Could you check a few things on this model? Use its own coordinates, in mm. Face numbers are marked on the shaded views. A direction names the side the tool comes from. Coordinates: 2 decimals unless noted, no trailing zeros. Loops run counter-clockwise (first coordinate to the right, second up) from the corner with the lowest first, then second, coordinate; pieces in that order, holes last. Notation, with made-up numbers: (-31.5, -31) - (-11.5, -31) arc R26 ccw to (-11.5, -13) - close; hole circle Ø2 at (10, 87.25). An arc over 180 degrees is marked (long way). Put each result on its own line as item: value. Start each with the question number.
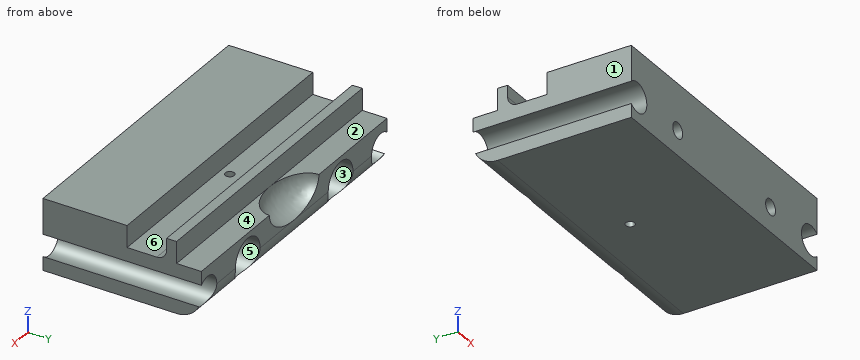
```python
from build123d import *

# Parameters (mm, degrees)
SKETCH2_W           = 18.288
SKETCH2_H           = 40.64
BOSS_EXTRUDE1_DEPTH = 76.2
CUT_EXTRUDE1_REACH  = 90.275
SKETCH3_W           = 5.588
SKETCH3_H           = 6.35
SKETCH3_H_2         = 10.16
CUT_EXTRUDE2_REACH  = 89.289
SKETCH4_R           = 1.143
CUT_EXTRUDE3_REACH  = 90.275
SKETCH5_R           = 2.032
SKETCH6_R           = 5.08
CUT_EXTRUDE4_DEPTH  = 15.24
FILLET1_R           = 6.35
FILLET2_R           = 2.54
SKETCH7_R           = 3.81
CUT_EXTRUDE5_DEPTH  = 89.275141297


with BuildPart() as part:
    # Sketch2 → Boss-Extrude1 (new body)
    with BuildSketch(Plane(origin=(0, 0, 0), x_dir=(0, 0, -1), z_dir=(1, 0, 0))):
        with Locations((9.144, 20.32)):
            Rectangle(SKETCH2_W, SKETCH2_H)
    extrude(amount=BOSS_EXTRUDE1_DEPTH)

    # Sketch3 → Cut-Extrude1 (cut, up to next)
    with BuildSketch(Plane.ZY, mode=Mode.PRIVATE) as cut_extrude1_sk1:
        with Locations((-2.794, 37.465)):
            Rectangle(SKETCH3_W, SKETCH3_H)
    cut_extrude1_tool1 = extrude(cut_extrude1_sk1.sketch, amount=-CUT_EXTRUDE1_REACH, mode=Mode.PRIVATE) & part.part
    # Sketch3 → Cut-Extrude1 (cut, up to next)
    with BuildSketch(Plane.ZY, mode=Mode.PRIVATE) as cut_extrude1_sk2:
        with Locations((-2.794, 26.67)):
            Rectangle(SKETCH3_W, SKETCH3_H_2)
    cut_extrude1_tool2 = extrude(cut_extrude1_sk2.sketch, amount=-CUT_EXTRUDE1_REACH, mode=Mode.PRIVATE) & part.part
    add(cut_extrude1_tool1.solids().sort_by_distance((0, 37.465, -2.794))[0], mode=Mode.SUBTRACT)
    add(cut_extrude1_tool2.solids().sort_by_distance((0, 26.67, -2.794))[0], mode=Mode.SUBTRACT)

    # Sketch4 → Cut-Extrude2 (cut, up to next)
    with BuildSketch(Plane.XY.offset(-5.588), mode=Mode.PRIVATE) as cut_extrude2_sk1:
        with Locations((38.1, 24.13)):
            Circle(SKETCH4_R)
    cut_extrude2_tool1 = extrude(cut_extrude2_sk1.sketch, amount=-CUT_EXTRUDE2_REACH, mode=Mode.PRIVATE) & part.part
    add(cut_extrude2_tool1.solids().sort_by_distance((38.1, 24.13, -5.588))[0], mode=Mode.SUBTRACT)

    # Sketch5 → Cut-Extrude3 (cut, up to next)
    with BuildSketch(Plane(origin=(0, 40.64, 0), x_dir=(1, 0, 0), z_dir=(0, 1, 0)), mode=Mode.PRIVATE) as cut_extrude3_sk1:
        with Locations(Location((57.15, 11.938, 0), (0, 0, 270))):
            Circle(SKETCH5_R)
    cut_extrude3_tool1 = extrude(cut_extrude3_sk1.sketch, amount=-CUT_EXTRUDE3_REACH, mode=Mode.PRIVATE) & part.part
    # Sketch5 → Cut-Extrude3 (cut, up to next)
    with BuildSketch(Plane(origin=(0, 40.64, 0), x_dir=(1, 0, 0), z_dir=(0, 1, 0)), mode=Mode.PRIVATE) as cut_extrude3_sk2:
        with Locations(Location((19.05, 11.938, 0), (0, 0, 270))):
            Circle(SKETCH5_R)
    cut_extrude3_tool2 = extrude(cut_extrude3_sk2.sketch, amount=-CUT_EXTRUDE3_REACH, mode=Mode.PRIVATE) & part.part
    add(cut_extrude3_tool1.solids().sort_by_distance((57.15, 40.64, -11.938))[0], mode=Mode.SUBTRACT)
    add(cut_extrude3_tool2.solids().sort_by_distance((19.05, 40.64, -11.938))[0], mode=Mode.SUBTRACT)

    # Sketch6 → Cut-Extrude4 (cut)
    with BuildSketch(Plane(origin=(0, 40.64, 0), x_dir=(1, 0, 0), z_dir=(0, 1, 0))):
        with Locations(Location((19.05, 11.938, 0), (0, 0, 270))):
            Circle(SKETCH6_R)
        with Locations(Location((57.15, 11.938, 0), (0, 0, 270))):
            Circle(SKETCH6_R)
    extrude(amount=-CUT_EXTRUDE4_DEPTH, mode=Mode.SUBTRACT)

    # Fillet1
    # the kernel refuses this fillet: 6.35 mm, written as the material it takes off along each edge
    with BuildSketch(Plane(origin=(-15.875, 40.64, -18.288), x_dir=(0, -1, 0), z_dir=(1, 0, 0))) as fillet1_piece_1:
        with BuildLine():
            CenterArc((FILLET1_R, -FILLET1_R), FILLET1_R, 90, 90)
            Line((0, -FILLET1_R), (0, 0))
            Line((0, 0), (FILLET1_R, 0))
        make_face()
    extrude(amount=107.95, mode=Mode.SUBTRACT)

    # Fillet2
    fillet2_edges = [part.edges().sort_by_distance(p)[0] for p in [
        (38.1, 31.75, -5.588),
    ]]
    fillet(fillet2_edges, radius=FILLET2_R)

    # Sketch7 → Cut-Extrude5 (cut, through all)
    with BuildSketch(Plane.XZ):
        with Locations((2.54, -11.938)):
            Circle(SKETCH7_R)
        with Locations((73.66, -11.938)):
            Circle(SKETCH7_R)
    extrude(amount=-CUT_EXTRUDE5_DEPTH, mode=Mode.SUBTRACT)

    # Sketch8 → Cut-Revolve3 (revolve, cut)
    with BuildSketch(Plane.XY.offset(-5.588)):
        with BuildLine():
            Line((27.94, 40.64), (48.26, 40.64))
            add(Edge.make_bspline(
                [(27.94, 40.64), (27.94, 34.29), (38.1, 34.29), (48.26, 34.29), (48.26, 40.64)],
                knots=[0, 0, 0, 1.570796327, 1.570796327, 3.141592654, 3.141592654, 3.141592654], degree=2, weights=[1, 0.707106781, 1, 0.707106781, 1]))
        make_face()
    revolve(axis=Axis((76.201, 40.64, -5.588), (-1, 0, 0)), mode=Mode.SUBTRACT)


solid = part.part
```
(1) For pin 1 Ø3.5 at (x, z) = (19.05, -11.938) entering from -Y; pin 2 Ø3 at (x, z) = (18.5, -11.5) entering from +Y; pin 3 Ø2 at (y, z) = (31, -6.5) entering from -X; pin 4 Ø2 at (y, z) = (36, -12.5) entering from +X, each with a flat end and sliding along its axis, tell me the tip position at first contact or that it passes through.
(2) If we mould it in two halves opening along Z, with no side actions, what happens to the marked faces 1, 2 and 3? For each: pulls with the +Z half, pulls with the -Z half, needs draft (parallel to the pull), parting line crosses it, or undercut.
(3) I want a section at D-D on x = 19.05. List the corners of the cut face in (y, z) for me.
(4) I need wall thicknesses on L1, parallel to Y at x = 6.5, z = -3; L2, parallel to X at y = 24, z = -6.75; L3, parallel to X at y = 35, z = -14.25. Which ranges of each line are inside material? Lowest first, please. Write a range as [from, to].
(5) I want a section at A-A on y = 24.13. List the corners of the cut face in (x, z) for me.
(6) Which directions (+Z, -Z, +X, -X, +Y, -Y) give clear straight access to the entire face, cutting with the end or side of a thin tool? Please do the marked faces 4, 5 and 6.
(7) I want a section at B-B on x = 73.66. List the corners of the cut face in (y, z) for me.
(8) I want a section at C-C on y = 19. List the corners of the cut face in (x, z) for me, and give its area (3 significant figures).
Answer sheet:
1. pin 1: passes through
1. pin 2: stops at y = 25.4
1. pin 3: stops at x = 0
1. pin 4: stops at x = 70.18
2. face 1: needs draft
2. face 2: pulls with the +Z half
2. face 3: undercut
3. outline: (0, -18.29) - (34.29, -18.29) arc R6.35 ccw to (38.1, -17.02) - (25.4, -17.02) - (25.4, -13.97) - (0, -13.97) - close; (0, -9.91) - (25.4, -9.91) - (25.4, -6.86) - (40.64, -6.86) - (40.64, -5.59) - (34.29, -5.59) - (34.29, 0) - (31.75, 0) - (31.75, -3.05) arc R2.54 cw to (29.21, -5.59) - (21.59, -5.59) - (21.59, 0) - (0, 0) - close
4. L1: y = [0, 21.59], [31.75, 34.29]
4. L2: x = [0, 36.96], [39.24, 76.2]
4. L3: x = [5.57, 14.53], [23.57, 52.63], [61.67, 70.63]
5. outline: (0, -18.29) - (36.96, -18.29) - (36.96, -5.59) - (0, -5.59) - (0, -9.1) arc R3.81 cw (long way) to (0, -14.78) - close; (39.24, -18.29) - (76.2, -18.29) - (76.2, -14.78) arc R3.81 cw (long way) to (76.2, -9.1) - (76.2, -5.59) - (39.24, -5.59) - close; hole circle Ø4.06 at (19.05, -11.94); hole circle Ø4.06 at (57.15, -11.94)
6. face 4: +Z, +X, -X, +Y
6. face 5: +Y
6. face 6: +Z, +X, -X
7. outline: (0, -18.29) - (34.29, -18.29) arc R6.35 ccw to (39.37, -15.75) - (0, -15.75) - close; (0, -8.13) - (40.64, -8.13) - (40.64, -5.59) - (34.29, -5.59) - (34.29, 0) - (31.75, 0) - (31.75, -3.05) arc R2.54 cw to (29.21, -5.59) - (21.59, -5.59) - (21.59, 0) - (0, 0) - close
8. outline: (0, -18.29) - (76.2, -18.29) - (76.2, -14.78) arc R3.81 cw (long way) to (76.2, -9.1) - (76.2, 0) - (0, 0) - (0, -9.1) arc R3.81 cw (long way) to (0, -14.78) - close; hole circle Ø4.06 at (19.05, -11.94); hole circle Ø4.06 at (57.15, -11.94)
8. area: 1,290 mm^2
